Here's how the part is built. I have some questions about the finished solid (model axes, mm). Face numbers are marked on the shaded views. A direction names the side the tool comes from. Round coordinates to 2 decimals unless told otherwise and drop trailing zeros. Order: outer loops, then holes, each group sorted by start corner. A loop starts at its lowest first (then second) coordinate and runs counter-clockwise, first axis right, second up. Notation, with made-up numbers: (15, 34.5) -> (51, 34.5) arc R24 ccw to (51, 65.5) -> close; hole circle Ø7 at (10, 37.5). An arc over 180 degrees is marked (long way). One line per item, written item: value.
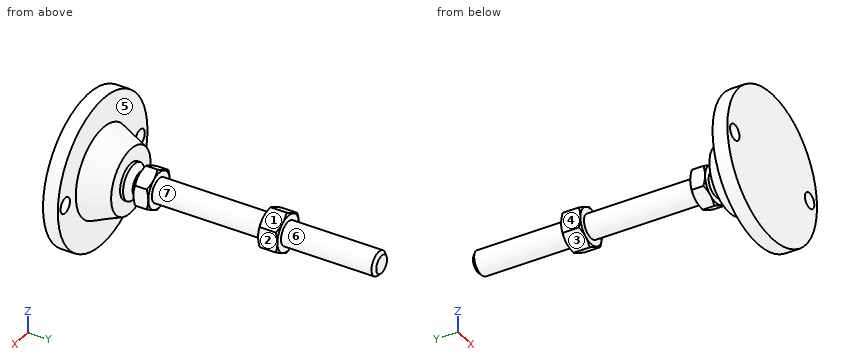
```python
from build123d import *

# Parameters (mm, degrees)
EXTRUDE_1_DEPTH     = 10
EXTRUDE_2_DEPTH     = 13
SKETCH_5_R          = 5.25
CUT_EXTRUDE_1_DEPTH = 11


with BuildPart() as part:
    # Эскиз1 → Повернуть1 (revolve)
    with BuildSketch(Plane.XY, mode=Mode.PRIVATE) as revolve_1_sk:
        Polygon((0, 0), (-50, 0), (-50, 10), (-30, 10), (-22, 29), (-12, 29), (-12, 31), (-8, 35), (-8, 38), (-8, 48), (-8, 196), (-6, 198), (0, 198), align=None)
    revolve(revolve_1_sk.sketch.rotate(Axis((0, 0, 0), (0, 1, 0)), 180), axis=Axis((0, 0, 0), (0, 1, 0)))  # turned: the seam where the file's is

    # Эскиз2 → Бобышка-Вытянуть1 (add)
    with BuildSketch(Plane(origin=(0, 38, 0), x_dir=(1, 0, 0), z_dir=(0, 1, 0))):
        Polygon((0, 13.856406461), (-12, 6.92820323), (-12, -6.92820323), (0, -13.856406461), (12, -6.92820323), (12, 6.92820323), align=None)
    extrude(amount=EXTRUDE_1_DEPTH)

    # Эскиз3 → Бобышка-Вытянуть2 (add)
    with BuildSketch(Plane(origin=(0, 122, 0), x_dir=(1, 0, 0), z_dir=(0, 1, 0))):
        Polygon((12, 6.92820323), (0, 13.856406461), (-12, 6.92820323), (-12, -6.92820323), (0, -13.856406461), (12, -6.92820323), align=None)
    extrude(amount=EXTRUDE_2_DEPTH)

    # Эскиз4 → Вырез-Повернуть2 (revolve, cut)
    with BuildSketch(Plane.XY, mode=Mode.PRIVATE) as cut_revolve_2_sk:
        Polygon((-23.258330249, 135), (-12, 135), (-23.258330249, 128.5), align=None)
        Polygon((-23.258330249, 122), (-23.258330249, 128.5), (-12, 122), align=None)
        Polygon((-20.660254038, 48), (-20.660254038, 43), (-12, 48), align=None)
        Polygon((-20.660254038, 43), (-20.660254038, 38), (-12, 38), align=None)
    revolve(cut_revolve_2_sk.sketch.rotate(Axis((0, 198, 0), (0, -1, 0)), 180), axis=Axis((0, 198, 0), (0, -1, 0)), mode=Mode.SUBTRACT)  # turned: the seam where the file's is

    # Эскиз5 → Вырез-Вытянуть1 (cut, through all)
    with BuildSketch(Plane(origin=(0, 10, 0), x_dir=(1, 0, 0), z_dir=(0, 1, 0))):
        with Locations(Location((-41.75, 0, 0), (0, 0, 180))):  # turned: the seam where the file's is
            Circle(SKETCH_5_R)
        with Locations(Location((41.75, 0, 0), (0, 0, 180))):  # turned: the seam where the file's is
            Circle(SKETCH_5_R)
    extrude(amount=-CUT_EXTRUDE_1_DEPTH, mode=Mode.SUBTRACT)


solid = part.part
```
Q1. I need wall thicknesses on line 1 along Y through (x, z) = (-11, -7); line 2 along Y through (x, z) = (2, -15); line 3 along Z through (x, y) = (-41, 2). Which ranges of each line are inside material? Lowest first, please.
Answers:
line 1: 0 to 29, 38.6 to 47.4, 122.6 to 134.4
line 2: 0 to 29
line 3: -28.62 to -5.2, 5.2 to 28.62
Q2. I want a section at A-A on x = -41.75. Write out the boundary of the cut face in (y, z).
Answers:
outline: (0, -27.51) -> (10, -27.51) -> (10, -5.25) -> (0, -5.25) -> close; (0, 5.25) -> (10, 5.25) -> (10, 27.51) -> (0, 27.51) -> close
Q3. For P1, Ø6.5, axis at y = 129.5, z = 2.5, coming from the +X side; P2, Ø9.5, axis at x = -41.75, z = 0, coming from the +Y side; P3, Ø4, axis at x = 1, y = 139, coming from the -Z side; P4, Ø14.5, axis at y = 131.5, z = 1, coming from the -X side, each with a flat end and sliding along its axis, tell me the tip position at first contact or that it passes through.
Answers:
P1: x = 12
P2: through
P3: z = -8
P4: x = -12
Q4. I want a section at B-B on y = 43. Write out the boundary of the cut face in (x, z), then the cut area to 3 significant figures.
Answers:
outline: (-12, -6.93) -> (0, -13.86) -> (12, -6.93) -> (12, 6.93) -> (0, 13.86) -> (-12, 6.93) -> close
area: 499 mm2
Q5. I want a section at D-D on y = 176.5. Write out the boundary of the cut face in (x, z), then the cut area to 3 significant figures.
Answers:
outline: circle Ø16 at (0, 0)
area: 201 mm2
Q6. I want a section at C-C on z = -34. Write out the boundary of the cut face in (x, y).
Answers:
outline: (-36.66, 0) -> (36.66, 0) -> (36.66, 10) -> (-36.66, 10) -> close
Q7. If we mould it in two halves opening along Y, with no side actions, what happens to the marked faces 5, 6 and 7? For each: pulls with the +Y half, pulls with the -Y half, needs draft (parallel to the pull), parting line crosses it, or undercut.
Answers:
face 5: pulls with the +Y half
face 6: needs draft
face 7: undercut
Q8. Which directions (+Z, -Z, +X, -X, +Y, -Y) give clear straight access to the entire face, cutting with the end or side of a thin tool? Please do the marked faces 1, 2, 3 and 4.
Answers:
face 1: +Z, +X, +Y
face 2: +Z, -Z, +X, +Y
face 3: -Z, -X, +Y
face 4: +Z, -Z, -X, +Y
